Here's how the part is built. I have some questions about the finished solid (model axes, mm). A direction names the side the tool comes from. Round coordinates to 2 decimals unless told otherwise and drop trailing zeros. Write each loop counter-clockwise with the first axis right and the second up, starting at its lowest first coordinate (ties: lowest second). Pieces come first, ordered by that corner, then holes. Notation, with made-up numbers: (-27.5, 3.25) -> (25.5, 3.25) arc R32 cw to (25.5, 36.25) -> close; hole circle Ø1 at (-13, -25). An arc over 180 degrees is marked (long way). Put each result on its own line as item: value. Start each with the question number.
1. Suppose I cut it at B-B (y = -180.5). Please give me the cut outline in (x, z).
2. For pin 1 (12 mm diameter, centred on y = -43, z = -534.5, fed in from -X); pin 2 (8 mm diameter, centred on x = 4, y = -222.5, fed in from +Z), each with a flat end and sliding along its axis, tell me the tip position at first contact or that it passes through.
3. Suppose I cut it at C-C (y = -69.5). Please give me the cut outline in (x, z).
4. Suppose I cut it at A-A (x = 14.25). Please give me the cut outline in (y, z).
5. I need wall thicknesses on probe 1 along Z at (x, y) = (2.5, -97); probe 2 along Z at (x, y) = (4, -75.5). Which ranges of each line are inside material? Lowest first, please. Write a range as from..to.
6. Which directions (+Z, -Z, +X, -X, +Y, -Y) give clear straight access to the entire face, cutting with the end or side of a thin tool? Please do faces 1 (the face through (9, -37, 0)), 2 (the face through (9, -212, 0)), 3 (the face through (8.874, -30.071, -591.484)).
```python
from build123d import *

# Parameters (mm, degrees)
BOSS_EXTRUDE1_DEPTH = 18


with BuildPart() as part:
    # Sketch1 → Boss-Extrude1 (new body)
    with BuildSketch(Plane(origin=(0, 0, 0), x_dir=(0, 0, -1), z_dir=(1, 0, 0))):
        with BuildLine():
            Line((0, -175), (0, -250))
            Line((0, -250), (620, -250))
            Line((620, -250), (620, -100))
            ThreePointArc((620, -100), (590.710678119, -29.289321881), (520, 0))
            Line((520, 0), (0, 0))
            Line((0, 0), (0, -75))
            Line((0, -75), (-18, -75))
            Line((-18, -75), (-18, -175))
            Line((-18, -175), (0, -175))
        make_face()
    extrude(amount=BOSS_EXTRUDE1_DEPTH)


solid = part.part
```
Verdict:
1. outline: (0, -620) -> (18, -620) -> (18, 0) -> (0, 0) -> close
2. pin 1: stops at x = 0
2. pin 2: stops at z = 0
3. outline: (0, -615.24) -> (18, -615.24) -> (18, 0) -> (0, 0) -> close
4. outline: (-250, -620) -> (-100, -620) arc R100 ccw to (0, -520) -> (0, 0) -> (-75, 0) -> (-75, 18) -> (-175, 18) -> (-175, 0) -> (-250, 0) -> close
5. probe 1: z = -619.95..18
5. probe 2: z = -616.95..18
6. face 1: +Z, +X, -X, +Y
6. face 2: +Z, +X, -X, -Y
6. face 3: -Z, +X, -X, +Y
